Work out the finished part from the listing and answer in its coordinate system (mm). Give positions to 0.01 mm unless a question says otherwise; leave off trailing zeros. Loops run counter-clockwise (first coordinate to the right, second up) from the corner with the lowest first, then second, coordinate; pieces in that order, holes last. Notation, with made-up numbers: M -12.75,-32 L 24.25,-32 A25 cw 24.25,-5 Z; hole C 87,70 d2. An arc over 180 degrees is marked long. Write item = value, one per line. Start each with the question number.
1. Consider L1, parallel to Z at x = -4.5, y = 1.75; L2, parallel to Y at x = 0, z = 269.25; L3, parallel to Y at x = -0.25, z = 79. Determine where each line is inside the solid, lowest interval first. Write a range as [from, to].
2. Flat-ended cylindrical pins translate along their axes: pin 1 Ø2 at (y, z) = (-5.5, 118) entering from +X; pin 2 Ø4 at (x, z) = (-5.5, 153.5) entering from -Y; pin 3 Ø6 at (y, z) = (5.5, 57.5) entering from +X. Find the tip coordinate at first contact, or state that the pin passes through.
3. Section A-A on z = 188 is taken. Determine the outline of the cut face in (x, y), plus the area to 3 significant figures.
```python
from build123d import *

# Parameters (mm, degrees)
SKETCH1_R           = 7.5
BOSS_EXTRUDE1_DEPTH = 242
SKETCH2_R           = 4
BOSS_EXTRUDE2_DEPTH = 30
SKETCH3_R           = 4
BOSS_EXTRUDE3_DEPTH = 20
SKETCH4_R           = 1.5
CUT_EXTRUDE1_DEPTH  = 8


with BuildPart() as part:
    # Sketch1 → Boss-Extrude1 (new body)
    with BuildSketch(Plane.XY):
        Circle(SKETCH1_R)
    extrude(amount=BOSS_EXTRUDE1_DEPTH)

    # Sketch2 → Boss-Extrude2 (add)
    with BuildSketch(Plane.XY.offset(242)):
        Circle(SKETCH2_R)
    extrude(amount=BOSS_EXTRUDE2_DEPTH)

    # Sketch3 → Boss-Extrude3 (add)
    with BuildSketch(Plane(origin=(0, 0, 0), x_dir=(-1, 0, 0), z_dir=(0, 0, -1))):
        Circle(SKETCH3_R)
    extrude(amount=BOSS_EXTRUDE3_DEPTH)

    # Sketch4 → Cut-Extrude1 (cut)
    with BuildSketch(Plane.XY.offset(272)):
        Circle(SKETCH4_R)
    extrude(amount=-CUT_EXTRUDE1_DEPTH, mode=Mode.SUBTRACT)


solid = part.part
```
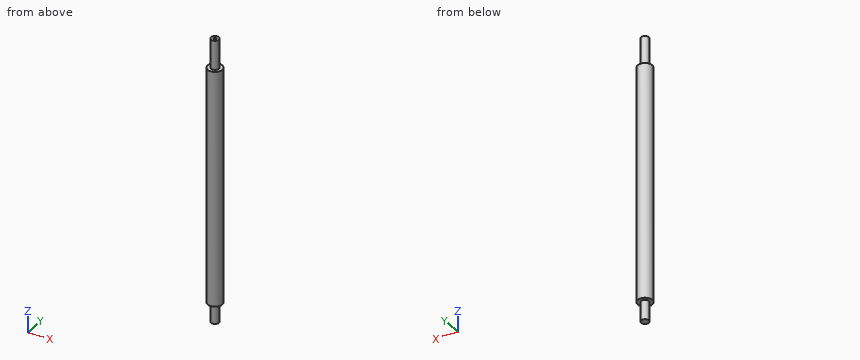
Verdict:
q1.L1 = [0, 242]
q1.L2 = [-4, -1.5], [1.5, 4]
q1.L3 = [-7.5, 7.5]
q2.pin_1 = 6
q2.pin_2 = -6.63
q2.pin_3 = 7.07
q3.outline = C 0,0 d15
q3.area = 177 mm2
